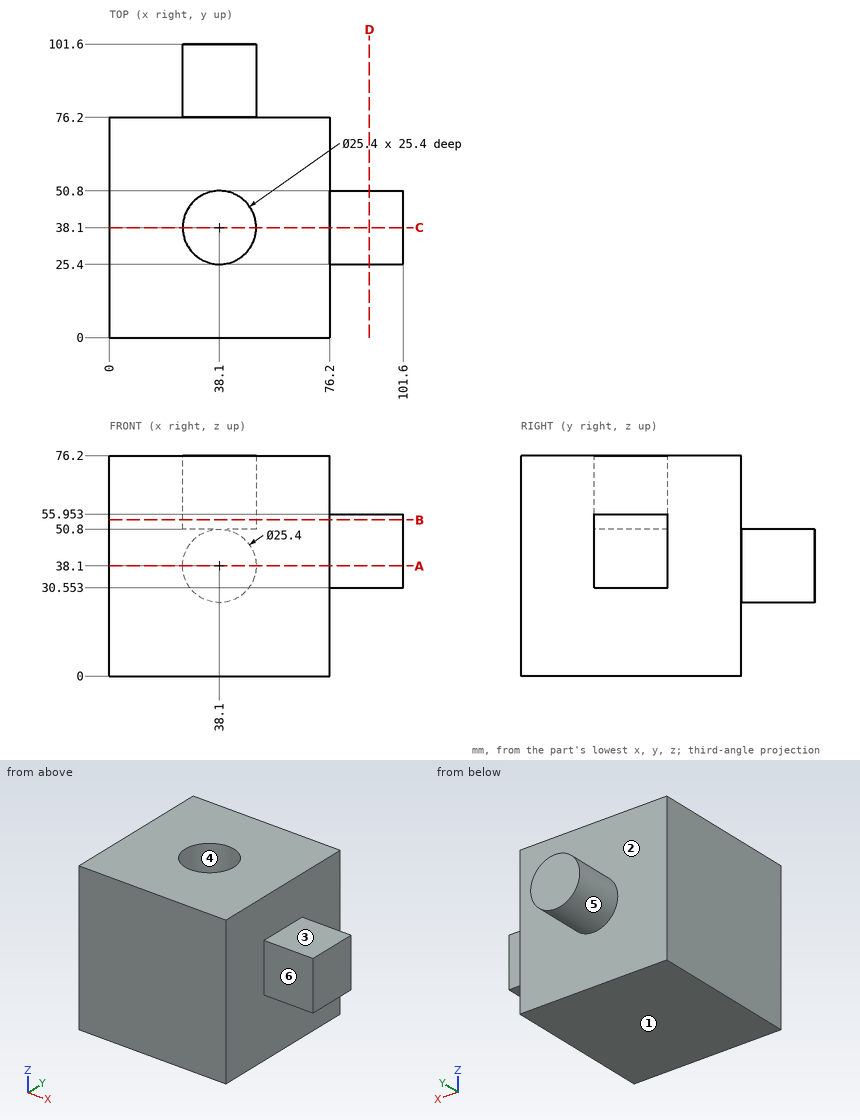
Geometry check sheet. Reference: drawing and pictorial views, mm from the part's lowest x, y, z. A direction names the side the tool comes from. Give positions to 0.01 mm unless a question says otherwise; leave off trailing zeros. Loops run counter-clockwise (first coordinate to the right, second up) from the corner with the lowest first, then second, coordinate; pieces in that order, holes last. Notation, with made-up numbers: (14, 77) - (70, 77) arc R25 cw to (70, 100) - close; hole circle Ø6 at (-23.5, 5.5). An arc over 180 degrees is marked (long way). One line per question, with ' | ' between items. Start each with the question number.
1. Set-up check for the marked faces 1, 2 and 3: record each of +Z, -Z, +X, -X, +Y, -Y from which the full face is reachable in a straight line by a thin tool's end or side.
2. Material ranges on line 1 along Y through (x, z) = (38, 68); line 2 along Y through (x, z) = (7, 62), recorded low to high. Write a range as [from, to].
3. Cross-section at A-A, the plane z = 38.1. Enter the section's corners in (x, y), plus the area to 3 significant figures.
4. Cross-section at D-D, the plane x = 90. Enter the section's corners in (y, z).
5. Gauge pin test, flat ends, axial feed: pin 1 Ø4 at (x, z) = (63.5, 31) entering from +Y; pin 2 Ø3 at (x, y) = (86, 48.5) entering from +Z; pin 3 Ø20.5 at (x, y) = (36, 35.5) entering from +Z; pin 4 Ø4 at (y, z) = (56, 47) entering from +X. Record the tip position at first contact, or that the pin passes through.
6. Draft check along X on the marked faces 4, 5 and 6. Enter one of: released by +X, released by -X, zero draft, split by the parting line, or undercut.
7. Cross-section at B-B, the plane z = 54. Enter the section's corners in (x, y), plus the area to 4 significant figures.
8. Cross-section at C-C, the plane y = 38.1. Enter the section's corners in (x, z).
Check result:
1) face 1: -Z, +X, -X, +Y, -Y | face 2: +Y | face 3: +Z, +X, +Y, -Y
2) line 1: y = [0, 25.4], [50.8, 76.2] | line 2: y = [0, 76.2]
3) outline: (0, 0) - (76.2, 0) - (76.2, 25.4) - (101.6, 25.4) - (101.6, 50.8) - (76.2, 50.8) - (76.2, 76.2) - (50.8, 76.2) - (50.8, 101.6) - (25.4, 101.6) - (25.4, 76.2) - (0, 76.2) - close | area: 7,100 mm2
4) outline: (25.4, 30.55) - (50.8, 30.55) - (50.8, 55.95) - (25.4, 55.95) - close
5) pin 1: stops at y = 76.2 | pin 2: stops at z = 55.95 | pin 3: stops at z = 76.2 | pin 4: stops at x = 76.2
6) face 4: undercut | face 5: split by the parting line | face 6: zero draft
7) outline: (0, 0) - (76.2, 0) - (76.2, 25.4) - (101.6, 25.4) - (101.6, 50.8) - (76.2, 50.8) - (76.2, 76.2) - (0, 76.2) - close; hole circle Ø25.4 at (38.1, 38.1) | area: 5,945 mm2
8) outline: (0, 0) - (76.2, 0) - (76.2, 30.55) - (101.6, 30.55) - (101.6, 55.95) - (76.2, 55.95) - (76.2, 76.2) - (50.8, 76.2) - (50.8, 50.8) - (25.4, 50.8) - (25.4, 76.2) - (0, 76.2) - close
